Here's how the part is built. I have some questions about the finished solid (model axes, mm). Face numbers are marked on the shaded views. A direction names the side the tool comes from. Coordinates: 2 decimals unless noted, no trailing zeros. Loops run counter-clockwise (first coordinate to the right, second up) from the corner with the lowest first, then second, coordinate; pieces in that order, holes last. Notation, with made-up numbers: (-26.5, -15) -> (-14.5, -15) arc R33 ccw to (-14.5, 16) -> close; hole circle Ø6 at (43, -34.5). An arc over 180 degrees is marked (long way). Use CSV: the item, a comma, the result in double quotes. Start each with the question number.
from build123d import *

# Parameters (mm, degrees)
SKETCH1_W                = 11
SKETCH1_H                = 5.3
BOSS_EXTRUDE1_DEPTH      = 2.9
SKETCH2_W                = 7.81
SKETCH2_H                = 2.5
BOSS_EXTRUDE2_DEPTH      = 0.7
BOSS_EXTRUDE3_DEPTH      = 1.6
BOSS_EXTRUDE3_DEPTH_BACK = 3.65
SKETCH3_R                = 0.25
CHAMFER1_SIZE            = 0.08
FILLET1_R                = 2.65
FILLET2_R                = 1.22


with BuildPart() as part:
    # Sketch1 → Boss-Extrude1 (new body)
    with BuildSketch(Plane(origin=(0, 0, 0), x_dir=(1, 0, 0), z_dir=(0, 1, 0))):
        with Locations((1.596774194, -1.130364656)):
            Rectangle(SKETCH1_W, SKETCH1_H)
    extrude(amount=BOSS_EXTRUDE1_DEPTH)

    # Sketch2 → Boss-Extrude2 (add)
    with BuildSketch(Plane(origin=(0, 2.9, 0), x_dir=(1, 0, 0), z_dir=(0, 1, 0))):
        with Locations((1.596774194, -1.130364656)):
            Rectangle(SKETCH2_W, SKETCH2_H)
    extrude(amount=BOSS_EXTRUDE2_DEPTH)

    # Sketch3 → Boss-Extrude3 (add, two sides: drawn at the far end of the back side and taken through both)
    with BuildSketch(Plane.XZ.offset(-BOSS_EXTRUDE3_DEPTH_BACK)):
        with Locations(Location((1.596774194, 1.130364656, 0), (0, 0, 90))):
            Circle(SKETCH3_R)
        with Locations(Location((3.096774194, 1.130364656, 0), (0, 0, 90))):
            Circle(SKETCH3_R)
        with Locations(Location((4.596774194, 1.130364656, 0), (0, 0, 90))):
            Circle(SKETCH3_R)
        with Locations(Location((0.096774194, 1.130364656, 0), (0, 0, 90))):
            Circle(SKETCH3_R)
        with Locations(Location((-1.403225806, 1.130364656, 0), (0, 0, 90))):
            Circle(SKETCH3_R)
    extrude(amount=BOSS_EXTRUDE3_DEPTH + BOSS_EXTRUDE3_DEPTH_BACK)

    # Chamfer1
    chamfer1_edges = [part.edges().sort_by_distance(p)[0] for p in [
        (1.596774194, -1.6, 0.880364656),
        (3.096774194, -1.6, 0.880364656),
        (4.596774194, -1.6, 0.880364656),
        (0.096774194, -1.6, 0.880364656),
        (-1.403225806, -1.6, 0.880364656),
    ]]
    chamfer(chamfer1_edges, length=CHAMFER1_SIZE)

    # Fillet1
    fillet1_edges = [part.edges().sort_by_distance(p)[0] for p in [
        (-3.903225806, 1.45, -1.519635344),
        (-3.903225806, 1.45, 3.780364656),
        (7.096774194, 1.45, 3.780364656),
        (7.096774194, 1.45, -1.519635344),
    ]]
    fillet(fillet1_edges, radius=FILLET1_R - 0.0001)  # a hair under: the kernel refuses the full size

    # Fillet2
    fillet2_edges = [part.edges().sort_by_distance(p)[0] for p in [
        (-2.308225806, 3.25, -0.119635344),
        (-2.308225806, 3.25, 2.380364656),
        (5.501774194, 3.25, 2.380364656),
        (5.501774194, 3.25, -0.119635344),
    ]]
    fillet(fillet2_edges, radius=FILLET2_R)


solid = part.part
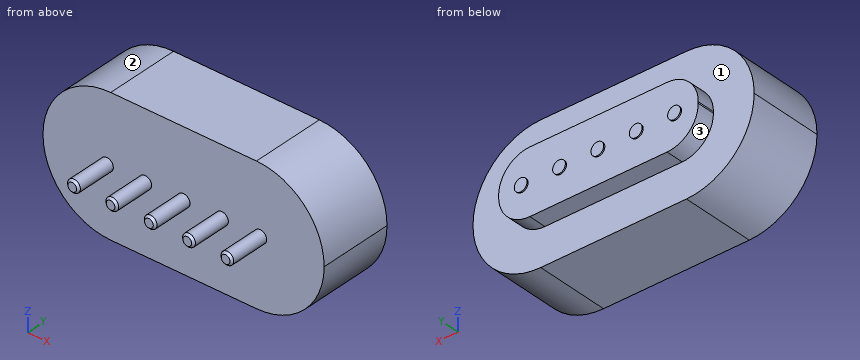
1) I want a section at D-D, the plane z = -0.3. Please give me the cut outline in (x, y).
2) I want a section at B-B, the plane y = -0.5. Please give me the cut outline in (x, z), plus the area to 3 significant figures.
3) Which directions (+Z, -Z, +X, -X, +Y, -Y) give clear straight access to the entire face, cutting with the end or side of a thin tool? Please do the marked faces 1, 2 and 3.
4) Please list where these lines run through material, in increasing order: L1, parallel to Y at x = 3.5, z = 2.75; L2, parallel to Y at x = 4.25, z = 0.6; L3, parallel to Z at x = -1, y = 3.3. Write a range as [from, to].
5) I want a section at A-A, the plane x = 3.75. Please give me the cut outline in (y, z).
6) For P1, Ø2, axis at x = -1.5, z = 3, coming from the +Y side; P2, Ø1.5, axis at x = -2.5, y = 1, coming from the +Z side; P3, Ø0.8, axis at x = 1.5, y = 3.5, coming from the -Z side, each with a flat end and sliding along its axis, tell me the tip position at first contact or that it passes through.
Return value:
1,outline,"(-3.48, 0) -> (6.68, 0) -> (6.68, 2.9) -> (-3.48, 2.9) -> close"
2,outline,"circle Ø0.5 at (-1.4, 1.13); circle Ø0.5 at (0.1, 1.13); circle Ø0.5 at (1.6, 1.13); circle Ø0.5 at (3.1, 1.13); circle Ø0.5 at (4.6, 1.13)"
2,area,"0.982 mm²"
3,face 1,"+Y"
3,face 2,"+Z, -X, +Y, -Y"
3,face 3,"-Z, -X, +Y"
4,L1,"y = [0, 2.9]"
4,L2,"y = [0, 3.6]"
4,L3,"z = [-0.12, 2.38]"
5,outline,"(0, -1.52) -> (2.9, -1.52) -> (2.9, -0.12) -> (3.6, -0.12) -> (3.6, 2.38) -> (2.9, 2.38) -> (2.9, 3.78) -> (0, 3.78) -> close"
6,P1,"stops at y = 3.6"
6,P2,"stops at z = 3.73"
6,P3,"stops at z = -0.12"
